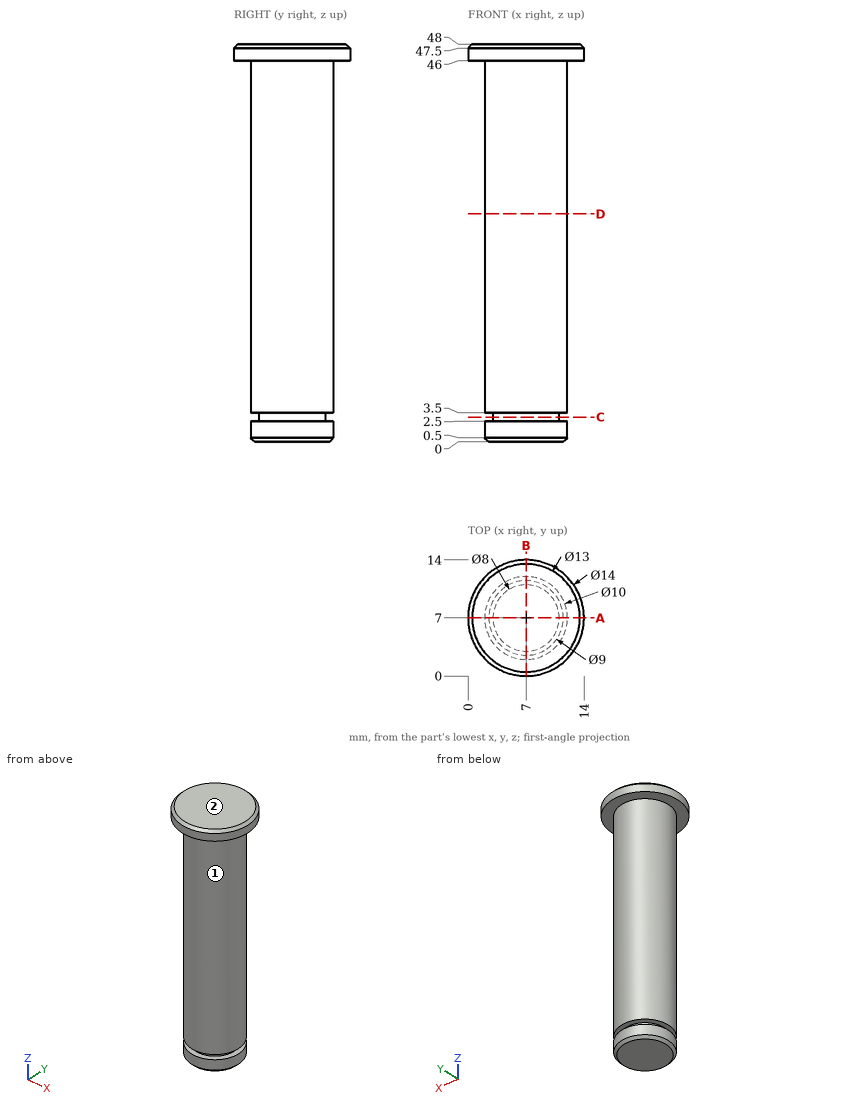
Here's the drawing with two shaded views (mm, measured from the low corner). I have some questions. A direction names the side the tool comes from. Coordinates: 2 decimals unless noted, no trailing zeros. Loops run counter-clockwise (first coordinate to the right, second up) from the corner with the lowest first, then second, coordinate; pieces in that order, holes last. Notation, with made-up numbers: M 80.25,30 L 91.25,30 A35 ccw 91.25,64 Z; hole C 15.5,-26 d11. An arc over 180 degrees is marked long. Return JSON: item names as keys, results as strings. Group by question number.
Item 1: I'm going to push flat-ended pins straight in: pin 1 Ø1.5 at (y, z) = (7, 9) entering from +X; pin 2 Ø1 at (x, z) = (6.5, 41.5) entering from -Y; pin 3 Ø1 at (x, z) = (4, 16) entering from +Y. Where does each tip first touch, or does it pass through?
Item 2: On a 3-axis mill with a long thin cutter (end or side, diameter ignored), from which of +Z, -Z, +X, -X, +Y, -Y can I reach the whole of each face in a straight line? I mean the marked faces 1 and 2. Say none if no direction works.
Item 3: Imagine slicing it at C-C (z = 3). Please give me the cut outline in (x, y), and give its area (3 significant figures).
Item 4: Imagine slicing it at A-A (y = 7). Please give me the cut outline in (x, z).
Item 5: If I drill on L1, parallel to Z at x = 2.25, y = 8.75; L2, parallel to X at y = 7.25, z = 12.5; L3, parallel to X at y = 4, z = 5.5, over which ranges is the centre line in solid material (lowest first)? Write a range as from..to.
Item 6: Imagine slicing it at D-D (z = 27.5). Please give me the cut outline in (x, y), and give its area (3 significant figures).
Verdict:
{
 "1": {"pin 1": "stops at x = 12", "pin 2": "stops at y = 2", "pin 3": "stops at y = 11.33"},
 "2": {"face 1": "-Z", "face 2": "+Z, +X, -X, +Y, -Y"},
 "3": {"outline": "C 7,7 d8", "area": "50.3 mm^2"},
 "4": {"outline": "M 0,46 L 2,46 L 2,3.5 L 3,3.5 L 3,2.5 L 2,2.5 L 2,0.5 L 2.5,0 L 11.5,0 L 12,0.5 L 12,2.5 L 11,2.5 L 11,3.5 L 12,3.5 L 12,46 L 14,46 L 14,47.5 L 13.5,48 L 0.5,48 L 0,47.5 Z"},
 "5": {"L1": "z = 46..48", "L2": "x = 2.01..11.99", "L3": "x = 3..11"},
 "6": {"outline": "C 7,7 d10", "area": "78.5 mm^2"}
}
